Model file for the job. Use its own axes, mm. Round coordinates to 2 decimals unless told otherwise and drop trailing zeros. Order: outer loops, then holes, each group sorted by start corner. A loop starts at its lowest first (then second) coordinate and runs counter-clockwise, first axis right, second up. Notation, with made-up numbers: (-38.5, 70) - (-24.5, 70) arc R19 ccw to (-24.5, 74) - close; hole circle Ø2 at (54.25, 8). An arc over 180 degrees is marked (long way). Write item = value, one per line.
Autodesk Inventor part; units mm, degrees
ref_plane "YZ Plane" through (0, 0, 0) normal (1, 0, 0) x (0, 1, 0)
ref_plane "XZ Plane" through (0, 0, 0) normal (0, 1, 0) x (-1, 0, 0)
ref_plane "XY Plane" through (0, 0, 0) normal (0, 0, 1) x (1, 0, 0)
sketch "Sketch1" plane through (0, 0, 0) normal (0, 0, 1) x (1, 0, 0)
  line L0 (3.175, 0) -> (3.175, 3.175)
  line L1 (3.175, 3.175) -> (-3.175, 3.175)
  line L2 (-3.175, 3.175) -> (-3.175, 0)
  line L3 (-5.08, 0) -> (-5.08, 5.08)
  line L4 (-5.08, 5.08) -> (5.08, 5.08)
  line L5 (5.08, 5.08) -> (5.08, 0)
  line L6 (5.08, 0) -> (3.175, 0)
  line L7 (-3.175, 0) -> (-5.08, 0)
  point P0 (0, 0)
  dimension "d0" = 10.16
  dimension "d1" = 5.08
extrude "Extrusion1" add sketch "Sketch1" along normal blind 368.3
sketch "Sketch2" plane through (-5.08, 5.08, 0) normal (0, 1, 0) x (1, 0, 0)
  circle A0 centre (5.08, -6.35) radius 1.9844
  circle A1 centre (5.08, -44.45) radius 1.9844
  circle A2 centre (5.08, -361.95) radius 1.9844
  circle A3 centre (5.08, -323.85) radius 1.9844
  point P0 (5.08, 0)
  dimension "d4" = 3.9688
  dimension "d5" = 3.9688
  dimension "d6" = 3.9688
  dimension "d7" = 3.9688
extrude "Extrusion2" cut sketch "Sketch2" against normal blind 368.3
sketch "Sketch3" plane through (0, 0, 0) normal (0, 0, -1) x (-1, 0, 0)
  line L0 (-5.08, 0) -> (-5.08, 5.08)
  line L1 (5.08, 5.08) -> (-5.08, 5.08)
  line L2 (-5.08, 5.08) -> (-5.08, 0)
  line L3 (-5.08, 0) -> (5.08, 0)
  line L4 (5.08, 0) -> (5.08, 5.08)
  point P0 (0, 0)
sketch "Sketch4" plane through (0, 0, 0) normal (0, 0, -1) x (-1, 0, 0)
  point P0 (0, 0)
extrude "Extrusion3" add sketch "Sketch3" along normal blind 1.778
sketch "Sketch5" plane through (-5.08, 5.08, 368.3) normal (0, 1, 0) x (1, 0, 0)
  circle A0 centre (5.08, 6.35) radius 1.9844
  circle A1 centre (5.08, 44.45) radius 1.9844
  circle A2 centre (5.08, 323.85) radius 1.9844
  circle A3 centre (5.08, 361.95) radius 1.9844
  circle A4 centre (5.08, 6.35) radius 5.08
  line L0 (10.16, 0) -> (10.16, 370.078)
  circle A5 centre (5.08, 44.45) radius 5.08
  circle A6 centre (5.08, 323.85) radius 5.08
  circle A7 centre (5.08, 361.95) radius 5.08
  point P0 (5.08, 368.3)
extrude "Extrusion4" add sketch "Sketch5" along normal blind 6.35
properties part number "hs_intake_cb_jig"
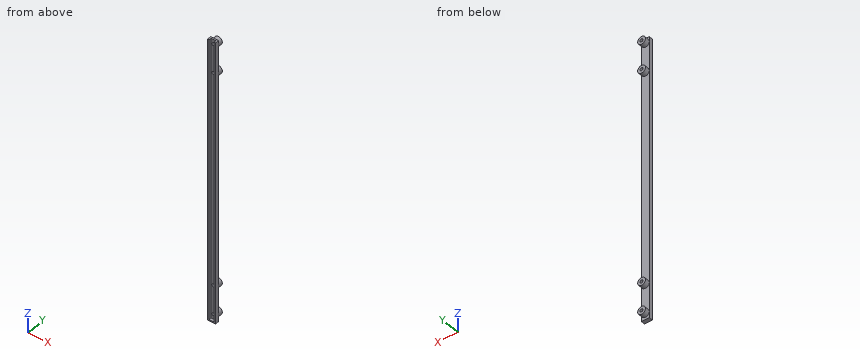
1) Cut at B-B (z = 304.5). Write the cut outline in (x, y) (3 decimals).
Conclusion:
outline = (-5.08, 0) - (-3.175, 0) - (-3.175, 3.175) - (3.175, 3.175) - (3.175, 0) - (5.08, 0) - (5.08, 5.08) - (-5.08, 5.08) - close
2) Flat gauge pins, fed straight in: pin 1 Ø1 at (x, y) = (3.5, 6.5) entering from -Z; pin 2 Ø3.5 at (x, z) = (0, 323.85) entering from -Y (1 decimal); pin 3 Ø5 at (x, z) = (0, 361.95) entering from -Y (3 decimals); pin 4 Ø1 at (x, y) = (4, 9.5) entering from -Z. Where does each tip first touch, or does it go through?
Conclusion:
pin_1 = 2.25
pin_2 = through
pin_3 = 3.175
pin_4 = 2.67
3) Cut at A-A (x = 0). Give the number of separate pieces and of enclosed holes in the cut face, and give its area (3 significant figures).
Conclusion:
separate_pieces = 5
enclosed_holes = 0
area = 838 mm^2
4) Wall check: line 1 along X through (y, z) = (2.5, 69) (3 decimals); line 2 along X through (y, z) = (9.5, 361.95); line 3 along Y through (x, z) = (-0.75, 91) (3 decimals). Give the ranges that are in metal, low to high.
Conclusion:
line_1 = -5.08 to -3.175, 3.175 to 5.08
line_2 = -5.08 to -1.98, 1.98 to 5.08
line_3 = 3.175 to 5.08
